```python
from build123d import *

# Parameters (mm, degrees)
F0_W     = 120
F0_H     = 60
F0_R     = 15
F1_DEPTH = 5
F2_R     = 5
F3_R     = 15
F4_DEPTH = 5
F5_W     = 20
F5_H     = 60
F6_DEPTH = 2.5


with BuildPart() as f1:
    # F0 (on Top) → F1 (new body)
    with BuildSketch(Plane.XY):
        Rectangle(F0_W, F0_H)
        with Locations((40, 0)):
            Circle(F0_R, mode=Mode.SUBTRACT)
    extrude(amount=F1_DEPTH)

    # F2
    f2_edges = [f1.edges().sort_by_distance(p)[0] for p in [
        (60, 30, 2.5),
        (60, -30, 2.5),
        (-60, 30, 2.5),
        (-60, -30, 2.5),
    ]]
    fillet(f2_edges, radius=F2_R)

    # F3 (on face) → F4 (join)
    with BuildSketch(Plane.XY.offset(5)):
        with Locations((-40, 0)):
            Circle(F3_R)
    extrude(amount=F4_DEPTH)

    # F5 (on face) → F6 (cut)
    with BuildSketch(Plane.XY.offset(5)):
        Rectangle(F5_W, F5_H)
    extrude(amount=-F6_DEPTH, mode=Mode.SUBTRACT)


solid = f1.part
```
Source: CAD feature listing. Evaluate the final solid. Frame: model axes, mm. A direction names the side the tool comes from. Coordinates: 2 decimals unless noted, no trailing zeros. Loops run counter-clockwise (first coordinate to the right, second up) from the corner with the lowest first, then second, coordinate; pieces in that order, holes last. Notation, with made-up numbers: (30, 24.5) -> (44, 24.5) arc R25 cw to (44, 42.5) -> close; hole circle Ø6 at (38.25, 12). An arc over 180 degrees is marked (long way). One line per item, written item: value. Start each with the question number.
Q1. Section query B-B, the plane y = -21. Return the cut outline in (x, z).
Q2. Section query C-C, the plane x = -40. Return the cut outline in (y, z).
Q3. Section query A-A, the plane x = 40. Return the cut outline in (y, z), and give its area (3 significant figures).
Q4. Line query: line 1 along Y through (x, z) = (40, 3.3); line 2 along Z through (x, y) = (26, 9.5); line 3 along Z through (x, y) = (3, 18.5). Output: solid intervals per line, ascending.
Q5. Set-up query: faces 5 (the face through (24, 0, 5)), 6 (the face through (-10, 0, 4)), 7 (the face through (-1, -30, 2)). Return all of +Z, -Z, +X, -X, +Y, -Y with unobstructed straight access to the full face (end or side cutting, diameter ignored); none if empty.
Q6. Section query D-D, the plane y = -7. Return the cut outline in (x, z).
Q7. Contact query for flat-ended pins moving along their axis: P1, Ø6, axis at x = 9.5, y = 1.5, coming from the +Z side; P2, Ø1.5, axis at x = -11, z = 7.5, coming from the -Y side. Output: stop coordinate, or through.
Q8. Mould query, pull axis X, two halves, no side actions, for faces 1 (the face through (25.015, 0.66, 2.465)), 2 (the face through (58, 29, 3)), 3 (the face through (-54.985, 0.66, 7.465)), 4 (the face through (-24, 0, 5)). Classes: pulls with the +X half, pulls with the -X half, needs draft (parallel to the pull), parting line crosses it, or undercut.
Results:
1. outline: (-60, 0) -> (60, 0) -> (60, 5) -> (10, 5) -> (10, 2.5) -> (-10, 2.5) -> (-10, 5) -> (-60, 5) -> close
2. outline: (-30, 0) -> (30, 0) -> (30, 5) -> (15, 5) -> (15, 10) -> (-15, 10) -> (-15, 5) -> (-30, 5) -> close
3. outline: (-30, 0) -> (-15, 0) -> (-15, 5) -> (-30, 5) -> close; (15, 0) -> (30, 0) -> (30, 5) -> (15, 5) -> close
3. area: 150 mm^2
4. line 1: -30 to -15, 15 to 30
4. line 2: 0 to 5
4. line 3: 0 to 2.5
5. face 5: +Z, +X, +Y, -Y
5. face 6: +Z, +Y, -Y
5. face 7: +Z, -Z, +X, -X, -Y
6. outline: (-60, 0) -> (26.73, 0) -> (26.73, 5) -> (10, 5) -> (10, 2.5) -> (-10, 2.5) -> (-10, 5) -> (-26.73, 5) -> (-26.73, 10) -> (-53.27, 10) -> (-53.27, 5) -> (-60, 5) -> close; (53.27, 0) -> (60, 0) -> (60, 5) -> (53.27, 5) -> close
7. P1: z = 5
7. P2: through
8. face 1: undercut
8. face 2: pulls with the +X half
8. face 3: parting line crosses it
8. face 4: needs draft
